from build123d import *

# Parameters (mm, degrees)
SKETCH_W        = 10
SKETCH_H        = 6
PAD_DEPTH       = 2.75
SKETCH001_R     = 1.65
HOLE_DEPTH      = 25
FILLET_R        = 3
FILLET001_R     = 1
POCKET_DEPTH    = 6.001
FILLET002_R     = 1.5
CHAMFER_SIZE    = 0.5
SKETCH002_R     = 1.65
PAD001_DEPTH    = 2.5
CHAMFER001_SIZE = 0.5
CHAMFER002_SIZE = 0.25


with BuildPart() as part:
    # Sketch → Pad (new body)
    with BuildSketch(Plane.XY):
        Rectangle(SKETCH_W, SKETCH_H)
    extrude(amount=PAD_DEPTH)

    # Sketch001 (on Face6 of Pad) → Hole (cut)
    with BuildSketch(Plane.XY.offset(2.75)):
        Circle(SKETCH001_R)
    extrude(amount=-HOLE_DEPTH, mode=Mode.SUBTRACT)

    # Fillet
    fillet_edges = [part.edges().sort_by_distance(p)[0] for p in [
        (-5, -3, 1.375),
        (5, 3, 1.375),
    ]]
    fillet(fillet_edges, radius=FILLET_R)

    # Fillet001
    fillet001_edges = [part.edges().sort_by_distance(p)[0] for p in [
        (-5, 3, 1.375),
        (5, -3, 1.375),
    ]]
    fillet(fillet001_edges, radius=FILLET001_R)

    # Sketch003 → Pocket (cut, through all)
    with BuildSketch(Plane.XZ.offset(3)):
        Polygon((-5, 1.25), (-2.5, 0), (-5, 0), align=None)
        Polygon((5, 1.25), (5, 0), (2.5, 0), align=None)
    extrude(amount=-POCKET_DEPTH, mode=Mode.SUBTRACT)

    # Fillet002
    fillet002_edges = [part.edges().sort_by_distance(p)[0] for p in [
        (-2.5, 0.02098, 0),
        (2.5, -0.02098, 0),
    ]]
    fillet(fillet002_edges, radius=FILLET002_R)

    # Chamfer
    chamfer_edges = [part.edges().sort_by_distance(p)[0] for p in [
        (-1, 3, 2.75),
        (0.072949, -3, 0),
    ]]
    chamfer(chamfer_edges, length=CHAMFER_SIZE)

    # Sketch002 (on Face5 of Hole) → Pad001 (join)
    with BuildSketch(Plane.XY.offset(1.75)):
        with BuildLine():
            ThreePointArc((0, 3), (-2.12132, 2.12132), (-3, 0))
            Line((-3, 0), (-3, -2))
            ThreePointArc((-3, -2), (-2.707107, -2.707107), (-2, -3))
            Line((-2, -3), (0, -3))
            ThreePointArc((0, -3), (2.12132, -2.12132), (3, 0))
            Line((3, 2), (3, 0))
            ThreePointArc((3, 2), (2.707107, 2.707107), (2, 3))
            Line((0, 3), (2, 3))
        make_face()
        Circle(SKETCH002_R, mode=Mode.SUBTRACT)
    extrude(amount=PAD001_DEPTH)

    # Chamfer001
    chamfer001_edges = [part.edges().sort_by_distance(p)[0] for p in [
        (-1, -3, 4.25),
    ]]
    chamfer(chamfer001_edges, length=CHAMFER001_SIZE)

    # Chamfer002
    chamfer002_edges = [part.edges().sort_by_distance(p)[0] for p in [
        (-1.65, 0, 0),
        (1.65, 0, 2.125),
        (-1.65, 0, 4.25),
    ]]
    chamfer(chamfer002_edges, length=CHAMFER002_SIZE)


solid = part.part
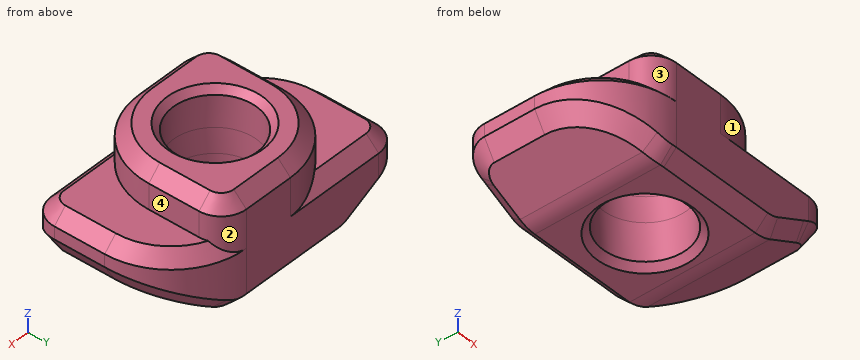
Here's how the part is built. I have some questions about the finished solid (model axes, mm). Face numbers are marked on the shaded views. A direction names the side the tool comes from. Give positions to 0.01 mm unless a question says otherwise; leave off trailing zeros. Write each loop counter-clockwise with the first axis right and the second up, starting at its lowest first coordinate (ties: lowest second). Pieces come first, ordered by that corner, then holes. Notation, with made-up numbers: (66.25, 62) -> (78.25, 62) arc R14 ccw to (78.25, 86) -> close; hole circle Ø10 at (65.25, -12). An arc over 180 degrees is marked (long way). Use one line per item in the form item = value. Start each with the question number.
1. On a 3-axis mill with a long thin cutter (end or side, diameter ignored), from which of +Z, -Z, +X, -X, +Y, -Y can I reach the whole of each face in a straight line? I mean the marked faces 1, 2, 3 and 4. Say none if no direction works.
2. If I drill on L1, parallel to Y at x = 0, z = 2.5; L2, parallel to Y at x = 1.25, z = 2.15; L3, parallel to X at y = -0.5, z = 3.3, over which ranges is the centre line in solid material (lowest first)?
3. Imagine slicing it at B-B on z = 2.6. List the corners of the cut face in (x, y) for me.
4. Will these pins go through, and if not, where does the flat tip stop? pin 1 Ø1.4 at (x, y) = (3.5, -1) entering from +Z; pin 2 Ø2 at (y, z) = (2, 3.5) entering from +X; pin 3 Ø3 at (x, y) = (0, 0) entering from -Z.
5. Imagine slicing it at A-A on z = 3.1. List the corners of the cut face in (x, y) for me.
Entries:
q1.face_1 = +Z, +X, -Y
q1.face_2 = +Z, +X, +Y
q1.face_3 = +Z, -X, -Y
q1.face_4 = +Z, +X, +Y, -Y
q2.L1 = -3 to -1.65, 1.65 to 3
q2.L2 = -3 to -1.08, 1.08 to 3
q2.L3 = -3 to -1.57, 1.57 to 2.96
q3.outline = (-4.65, 0) arc R2.65 ccw to (-2.86, -2.51) arc R1 ccw to (-2, -3) -> (0, -3) arc R3 ccw to (1.41, -2.65) -> (4, -2.65) arc R0.65 ccw to (4.65, -2) -> (4.65, 0) arc R2.65 ccw to (2.86, 2.51) arc R1 ccw to (2, 3) -> (0, 3) arc R3 ccw to (-1.41, 2.65) -> (-4, 2.65) arc R0.65 ccw to (-4.65, 2) -> close; hole circle Ø3.3 at (0, 0)
q4.pin_1 = 3.81
q4.pin_2 = 4.14
q4.pin_3 = through
q5.outline = (-3, -2) arc R1 ccw to (-2, -3) -> (0, -3) arc R3 ccw to (3, 0) -> (3, 2) arc R1 ccw to (2, 3) -> (0, 3) arc R3 ccw to (-3, 0) -> close; hole circle Ø3.3 at (0, 0)
